Check sheet for the modelled part. Datum: model origin and axes. Units: mm. A direction names the side the tool comes from. Give positions to 0.01 mm unless a question says otherwise; leave off trailing zeros. Write each loop counter-clockwise with the first axis right and the second up, starting at its lowest first coordinate (ties: lowest second). Pieces come first, ordered by that corner, then holes. Notation, with made-up numbers: (-18.5, -25.5) -> (-1.5, -25.5) arc R18 ccw to (-1.5, -6.5) -> close; hole circle Ø10 at (77, 36.5). An arc over 180 degrees is marked (long way). Use a Markdown table: item, result. Add a question column.
1. Cross-section at B-B (z = 52.5). Enter the section's corners in (x, y) (3 decimals), then the cut area to 3 significant figures.
2. Scan lines: probe 1 along Y at (x, z) = (0, 36) (3 decimals); probe 2 along X at (y, z) = (19, 50.5). Record each from-to range of solid material in increasing order. Write a range as [from, to].
3. Cross-section at D-D (z = 77). Enter the section's corners in (x, y) (3 decimals), then the cut area to 3 significant figures.
4. Release check for a two-part mould opening along Y. For faces 1 (the flat face through (-7, 11, 0)), 2 (the cylindrical face through (-0.28, 4.85, 53.97)), 3 (the cylindrical face through (-3.441, -15.497, 40.697)) record: released by +Y, released by -Y, zero draft, split by the parting line, or undercut.
5. Cross-section at C-C (x = -9). Enter the section's corners in (y, z).
6. Gauge pin test, flat ends, axial feed: P1, Ø6, axis at x = 12.5, z = 52.5, coming from the +Y side; P2, Ø5, axis at y = 9, z = 58, coming from the -X side; P3, Ø4, axis at x = 11, z = 58, coming from the -Y side; P4, Ø5, axis at x = 8.5, y = 18.5, coming from the +Z side. Record the tip position at first contact, or that the pin passes through.
7. Cross-section at A-A (x = 0). Enter the section's corners in (y, z) (3 decimals), then the cut area to 3 significant figures.
8. Set-up check for faces 4 (the flat face through (-1, 0, 54.5)), 5 (the cylindrical face through (0.28, 4.85, 28.58)), 6 (the flat face through (-7, 11, 82.55)), 7 (the cylindrical face through (-8.58, 24.95, 50.64)): record each of +Z, -Z, +X, -X, +Y, -Y from which the full face is reachable in a straight line by a thin tool's end or side.
from build123d import *

# Parameters (mm, degrees)
SKETCH1_R           = 15.875
SKETCH1_R_2         = 12.7
BOSS_EXTRUDE1_DEPTH = 82.55
SKETCH2_R           = 15.875
SKETCH2_R_2         = 12.7
BOSS_EXTRUDE2_DEPTH = 35.052


with BuildPart() as part:
    # Sketch1 → Boss-Extrude1 (new body)
    with BuildSketch(Plane.XY):
        Circle(SKETCH1_R)
        Circle(SKETCH1_R_2, mode=Mode.SUBTRACT)
    extrude(amount=BOSS_EXTRUDE1_DEPTH)

    # Sketch2 → Boss-Extrude2 (add)
    with BuildSketch(Plane(origin=(0, 0, 0), x_dir=(1, 0, 0), z_dir=(0, 1, 0))):
        with Locations((0, -41.275)):
            Circle(SKETCH2_R)
        with Locations(Location((0, -41.275, 0), (0, 0, 90))):
            Circle(SKETCH2_R_2, mode=Mode.SUBTRACT)
    extrude(amount=BOSS_EXTRUDE2_DEPTH)


solid = part.part
Worked answers:
| question | item | result |
|---|---|---|
| 1 | outline | (-11.226, 11.225) arc R15.875 ccw (long way) to (11.226, 11.225) -> (11.226, 35.052) -> (5.94, 35.052) -> (5.94, 14.722) arc R15.875 ccw to (-5.94, 14.722) -> (-5.94, 35.052) -> (-11.226, 35.052) -> close; hole (-11.226, 0) -> (-11.226, 5.939) arc R12.7 ccw (long way) to (11.226, 5.939) -> (11.226, 0) -> (5.94, 0) -> (5.94, 11.225) arc R12.7 ccw to (-5.94, 11.225) -> (-5.94, 0) -> close |
| 1 | area | 612 mm² |
| 2 | probe 1 | y = [-15.875, -12.7], [12.7, 15.875] |
| 2 | probe 2 | x = [-12.92, -8.73], [8.73, 12.92] |
| 3 | outline | circle Ø31.75 at (0, 0); hole circle Ø25.4 at (0, 0) |
| 3 | area | 285 mm² |
| 4 | face 1 | zero draft |
| 4 | face 2 | undercut |
| 4 | face 3 | split by the parting line |
| 5 | outline | (-13.08, 0) -> (-8.96, 0) -> (-8.96, 82.55) -> (-13.08, 82.55) -> close; (0, 28.2) -> (8.96, 28.2) -> (8.96, 0) -> (13.08, 0) -> (13.08, 28.2) -> (35.05, 28.2) -> (35.05, 32.31) -> (13.08, 32.31) -> (13.08, 50.24) -> (35.05, 50.24) -> (35.05, 54.35) -> (13.08, 54.35) -> (13.08, 82.55) -> (8.96, 82.55) -> (8.96, 54.35) -> (0, 54.35) -> (0, 50.24) -> (8.96, 50.24) -> (8.96, 32.31) -> (0, 32.31) -> close |
| 6 | P1 | stops at y = 35.05 |
| 6 | P2 | stops at x = -14.48 |
| 6 | P3 | stops at y = -13.08 |
| 6 | P4 | stops at z = 55.97 |
| 7 | outline | (-15.875, 0) -> (-12.7, 0) -> (-12.7, 82.55) -> (-15.875, 82.55) -> close; (0, 25.4) -> (12.7, 25.4) -> (12.7, 0) -> (15.875, 0) -> (15.875, 25.4) -> (35.052, 25.4) -> (35.052, 28.575) -> (15.875, 28.575) -> (15.875, 53.975) -> (35.052, 53.975) -> (35.052, 57.15) -> (15.875, 57.15) -> (15.875, 82.55) -> (12.7, 82.55) -> (12.7, 57.15) -> (0, 57.15) -> (0, 53.975) -> (12.7, 53.975) -> (12.7, 28.575) -> (0, 28.575) -> close |
| 7 | area | 727 mm² |
| 8 | face 4 | +Z, -Z |
| 8 | face 5 | none |
| 8 | face 6 | +Z, +X, -X, +Y, -Y |
| 8 | face 7 | +Y |
